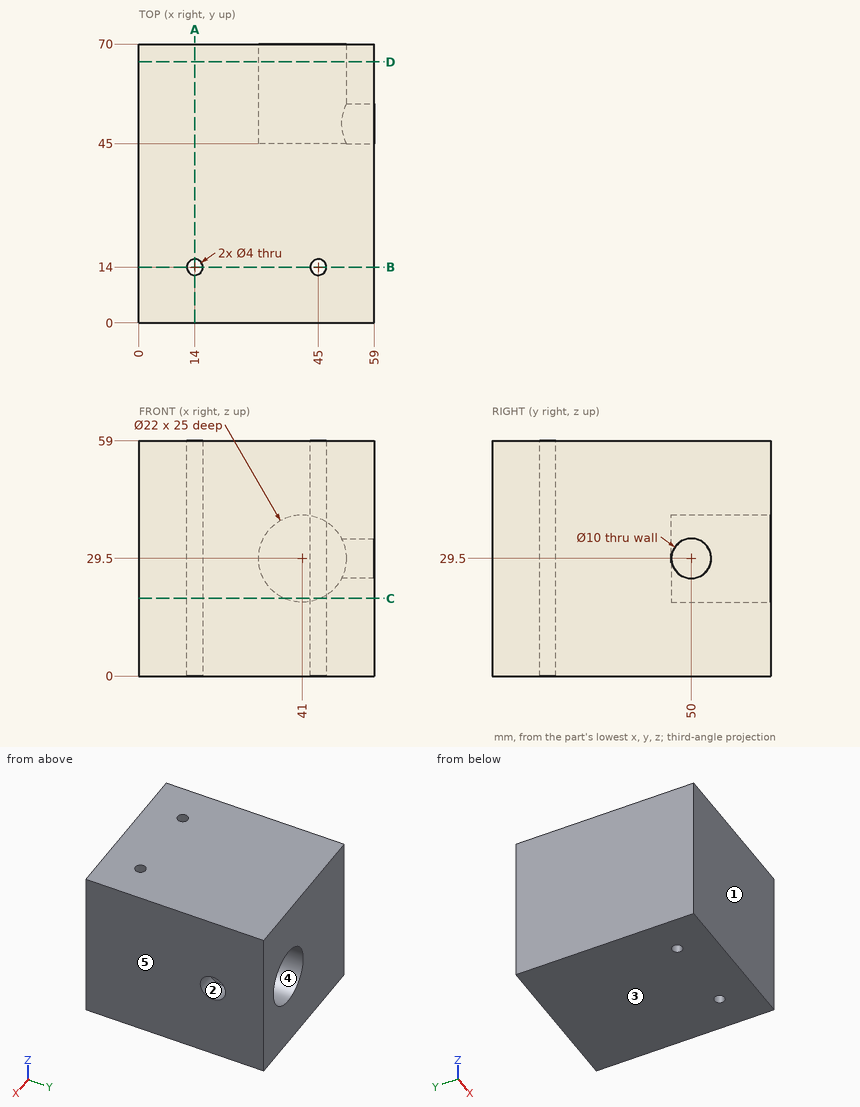
Job drawing, mm, ordinate dimensions from the low corner. One solid piece. A direction names the side the tool comes from. Give positions to 0.01 mm unless a question says otherwise; leave off trailing zeros. Write each loop counter-clockwise with the first axis right and the second up, starting at its lowest first coordinate (ties: lowest second). Pieces come first, ordered by that corner, then holes. Notation, with made-up numbers: (-11, -5) - (28, -5) arc R16 ccw to (28, -1) - close; hole circle Ø4 at (6, -14.5). An arc over 180 degrees is marked (long way). Use one line per item in the form item = value. Start each with the question number.
1. Band-saw the part on B-B on y = 14. Write the cut outline in (x, z).
2. Two-plate mould, pull along Z, no slides. Class the marked faces 1, 2 and 3: released by +Z, released by -Z, zero draft, split by the parting line, or undercut.
3. Band-saw the part on D-D on y = 65.5. Write the cut outline in (x, z), plus the area to 3 significant figures.
4. Probe line 1 (Y direction, x = 14, z = 34.5); line 2 (Z direction, x = 41, y = 58.25); line 3 (X direction, y = 58, z = 29). List the from-to ranges inside material, lowest first. Write a range as [from, to].
5. Band-saw the part on C-C on z = 19.5. Write the cut outline in (x, y).
6. Band-saw the part on A-A on x = 14. Write the cut outline in (y, z).
7. 3-axis set-ups, long thin cutter, end or side, ignore diameter. For the marked faces 4 and 5: which of +Z, -Z, +X, -X, +Y, -Y reach the whole face in a straight line?
Conclusion:
q1.outline = (0, 0) - (12, 0) - (12, 59) - (0, 59) - close; (16, 0) - (43, 0) - (43, 59) - (16, 59) - close; (47, 0) - (59, 0) - (59, 59) - (47, 59) - close
q2.face_1 = zero draft
q2.face_2 = undercut
q2.face_3 = released by -Z
q3.outline = (0, 0) - (59, 0) - (59, 59) - (0, 59) - close; hole circle Ø22 at (41, 29.5)
q3.area = 3,100 mm²
q4.line_1 = [0, 12], [16, 70]
q4.line_2 = [0, 18.5], [40.5, 59]
q4.line_3 = [0, 30.01], [51.99, 59]
q5.outline = (0, 0) - (59, 0) - (59, 70) - (45.58, 70) - (45.58, 45) - (36.42, 45) - (36.42, 70) - (0, 70) - close; hole circle Ø4 at (14, 14); hole circle Ø4 at (45, 14)
q6.outline = (0, 0) - (12, 0) - (12, 59) - (0, 59) - close; (16, 0) - (70, 0) - (70, 59) - (16, 59) - close
q7.face_4 = +Y
q7.face_5 = +Z, -Z, +X, +Y, -Y
